```python
from build123d import *

# Parameters (mm, degrees)
SKETCH_1_W          = 50
SKETCH_1_H          = 25
EXTRUDE_1_DEPTH     = 50
CUT_EXTRUDE_3_DEPTH = 62.23724357
FILLET_1_R          = 1.25
FILLET_2_R          = 0.5


with BuildPart() as part:
    # 草图1 → 拉伸1 (new body)
    with BuildSketch(Plane(origin=(0, 0, 0), x_dir=(1, 0, 0), z_dir=(0, 1, 0))):
        Rectangle(SKETCH_1_W, SKETCH_1_H)
    extrude(amount=EXTRUDE_1_DEPTH)

    # 草图3 → 切除-拉伸3 (cut, through all)
    with BuildSketch(Plane(origin=(0, 0, -12.5), x_dir=(-1, 0, 0), z_dir=(0, 0, -1))):
        Polygon((-19, 50), (-19, 47), (-22.2, 47), (-22.2, 8), (-19.625, 8), (-19.125, 40), (-18.525, 40), (-18.025, 8), (-15.975, 8), (-15.775, 40), (-15.175, 40), (-14.975, 8), (-12.625, 8), (-12.425, 50), (-11.825, 50), (-11.625, 8), (-9.275, 8), (-9.075, 50), (-8.475, 50), (-8.275, 8), (-5.925, 8), (-5.725, 50), (-5.125, 50), (-4.925, 8), (-2.575, 8), (-2.375, 50), (-1.775, 50), (-1.575, 8), (1.575, 8), (1.775, 50), (2.375, 50), (2.575, 8), (4.925, 8), (5.125, 50), (5.725, 50), (5.925, 8), (8.275, 8), (8.475, 50), (9.075, 50), (9.275, 8), (11.625, 8), (11.825, 50), (12.425, 50), (12.625, 8), (14.975, 8), (15.175, 40), (15.775, 40), (15.975, 8), (18.025, 8), (18.525, 40), (19.125, 40), (19.625, 8), (22.2, 8), (22.2, 47), (19, 47), (19, 50), (19, 55.346255007), (-19, 55.346255007), align=None)
    extrude(amount=-CUT_EXTRUDE_3_DEPTH, mode=Mode.SUBTRACT)

    # 圆角1
    # the kernel refuses this fillet: 1.25 mm, written as the material it adds along each edge
    with BuildSketch(Plane(origin=(-2.575, 8, -12.5), x_dir=(0.004761850772972935, 0.9999886623243365, 0), z_dir=(0, 0, 1)), Plane(origin=(-1.575, 8, -12.5), x_dir=(1, 0, 0), z_dir=(0, 0, 1)), Plane(origin=(1.575, 8, -12.5), x_dir=(0.004761850772973114, 0.9999886623243365, 0), z_dir=(0, 0, 1)), Plane(origin=(2.575, 8, -12.5), x_dir=(1, 0, 0), z_dir=(0, 0, 1)), Plane(origin=(4.925, 8, -12.5), x_dir=(0.004761850772972935, 0.9999886623243365, 0), z_dir=(0, 0, 1)), Plane(origin=(5.925, 8, -12.5), x_dir=(1, 0, 0), z_dir=(0, 0, 1)), Plane(origin=(8.275, 8, -12.5), x_dir=(0.004761850772972963, 0.9999886623243365, 0), z_dir=(0, 0, 1)), Plane(origin=(9.275, 8, -12.5), x_dir=(1, 0, 0), z_dir=(0, 0, 1)), Plane(origin=(11.625, 8, -12.5), x_dir=(0.004761850772972963, 0.9999886623243365, 0), z_dir=(0, 0, 1)), Plane(origin=(12.625, 8, -12.5), x_dir=(1, 0, 0), z_dir=(0, 0, 1)), Plane(origin=(-12.625, 8, -12.5), x_dir=(0.004761850772972963, 0.9999886623243365, 0), z_dir=(0, 0, 1)), Plane(origin=(-11.625, 8, -12.5), x_dir=(1, 0, 0), z_dir=(0, 0, 1)), Plane(origin=(-9.275, 8, -12.5), x_dir=(0.004761850772972963, 0.9999886623243365, 0), z_dir=(0, 0, 1)), Plane(origin=(-8.275, 8, -12.5), x_dir=(1, 0, 0), z_dir=(0, 0, 1)), Plane(origin=(-5.925, 8, -12.5), x_dir=(0.004761850772972935, 0.9999886623243365, 0), z_dir=(0, 0, 1)), Plane(origin=(-4.925, 8, -12.5), x_dir=(1, 0, 0), z_dir=(0, 0, 1))) as fillet_1_piece_1:
        with BuildLine():
            CenterArc((FILLET_1_R * 0.995249433042, FILLET_1_R), FILLET_1_R, 180.272834983, 89.727165017)
            Line((-FILLET_1_R * 0.00473922928203, FILLET_1_R * 0.995238149227), (0, 0))
            Line((0, 0), (FILLET_1_R * 0.995249433042, 0))
        make_face()
    extrude(amount=25)
    with BuildSketch(Plane(origin=(14.975, 8, -12.5), x_dir=(0.006249877933264038, 0.999980469322186, 0), z_dir=(0, 0, 1)), Plane(origin=(15.975, 8, -12.5), x_dir=(1, 0, 0), z_dir=(0, 0, 1)), Plane(origin=(-15.975, 8, -12.5), x_dir=(0.00624987793326402, 0.999980469322186, 0), z_dir=(0, 0, 1)), Plane(origin=(-14.975, 8, -12.5), x_dir=(1, 0, 0), z_dir=(0, 0, 1))) as fillet_1_piece_2:
        with BuildLine():
            CenterArc((FILLET_1_R * 0.993769531059, FILLET_1_R), FILLET_1_R, 180.358093959, 89.641906041)
            Line((-FILLET_1_R * 0.00621093826293, FILLET_1_R * 0.993750122067), (0, 0))
            Line((0, 0), (FILLET_1_R * 0.993769531059, 0))
        make_face()
    extrude(amount=25)
    with BuildSketch(Plane(origin=(18.025, 8, -12.5), x_dir=(0.015623093000541032, 0.9998779520346953, 0), z_dir=(0, 0, 1)), Plane(origin=(19.625, 8, -12.5), x_dir=(1, 0, 0), z_dir=(0, 0, 1)), Plane(origin=(-19.625, 8, -12.5), x_dir=(0.015623093000541032, 0.9998779520346953, 0), z_dir=(0, 0, 1)), Plane(origin=(-18.025, 8, -12.5), x_dir=(1, 0, 0), z_dir=(0, 0, 1))) as fillet_1_piece_3:
        with BuildLine():
            CenterArc((FILLET_1_R * 0.984497062863, FILLET_1_R), FILLET_1_R, 180.89517371, 89.10482629)
            Line((-FILLET_1_R * 0.0153808891719, FILLET_1_R * 0.984376906999), (0, 0))
            Line((0, 0), (FILLET_1_R * 0.984497062863, 0))
        make_face()
    extrude(amount=25)
    with BuildSketch(Plane(origin=(22.2, 8, -12.5), x_dir=(0, 1, 0), z_dir=(0, 0, 1)), Plane(origin=(-22.2, 8, -12.5), x_dir=(1, 0, 0), z_dir=(0, 0, 1))) as fillet_1_piece_4:
        with BuildLine():
            CenterArc((FILLET_1_R, FILLET_1_R), FILLET_1_R, 180, 90)
            Line((0, FILLET_1_R), (0, 0))
            Line((0, 0), (FILLET_1_R, 0))
        make_face()
    extrude(amount=25)

    # 圆角2
    fillet_2_edges = [part.edges().sort_by_distance(p)[0] for p in [
        (25, 50, 0),
        (22.2, 47, 0),
        (19, 47, 0),
        (19, 50, 0),
        (-19, 50, 0),
        (-25, 50, 0),
        (-19, 47, 0),
        (-22.2, 47, 0),
    ]]
    fillet(fillet_2_edges, radius=FILLET_2_R)


solid = part.part
```
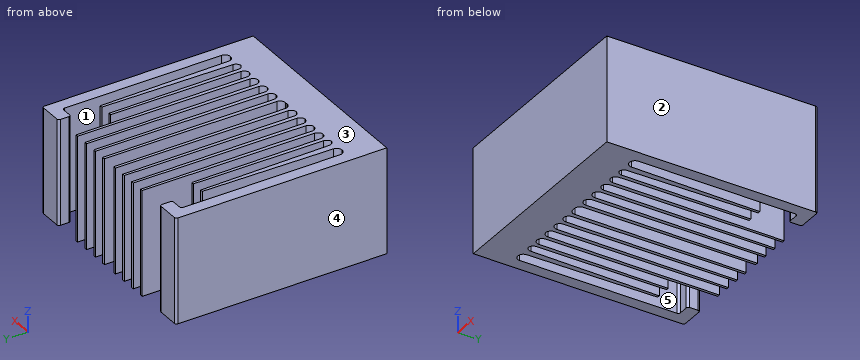
Can you work these out from the model? Positions are in its coordinate system, mm. Face numbers are marked on the shaded views. A direction names the side the tool comes from. Round coordinates to 2 decimals unless told otherwise and drop trailing zeros. One line per item, written item: value. Start each with the question number.
1. For pin 1 (10 mm diameter, centred on x = 9.5, z = 3, fed in from +Y); pin 2 (0.7 mm diameter, centred on x = 15.5, z = -2.5, fed in from +Y), each with a flat end and sliding along its axis, tell me the tip position at first contact or that it passes through.
2. If we mould it in two halves opening along X, with no side actions, what happens to the marked faces 3, 4 and 5? For each: pulls with the +X half, pulls with the -X half, needs draft (parallel to the pull), parting line crosses it, or undercut.
3. If I drill on probe 1 along Y at (x, z) = (-21, 10.75); probe 2 along Y at (x, z) = (0.5, -11.25); probe 3 along Y at (x, z) = (-3, 8), over which ranges is the centre line in solid material (lowest first)?
4. For the marked faces 1 and 2, which set-ups out of +Z, -Z, +X, -X, +Y, -Y let a thin tool reach every point of the face, with its end or its side?
5. If we section it at A-A, the plane y = 33.5: Give the number of separate pieces and of enclosed holes in the cut face, then the cut area to 3 significant figures.
Calculated:
1. pin 1: stops at y = 50
1. pin 2: stops at y = 40
2. face 3: needs draft
2. face 4: pulls with the -X half
2. face 5: undercut
3. probe 1: y = 0 to 8, 47 to 50
3. probe 2: y = 0 to 8.01
3. probe 3: y = 0 to 8.31
4. face 1: +Z, -Z
4. face 2: +Z, -Z, +X, +Y, -Y
5. separate pieces: 14
5. enclosed holes: 0
5. area: 366 mm²
